Here's the drawing with two shaded views (mm, measured from the low corner). I have some questions. Give positions to 0.01 mm unless a question says otherwise; leave off trailing zeros. Write each loop counter-clockwise with the first axis right and the second up, starting at its lowest first coordinate (ties: lowest second). Pieces come first, ordered by that corner, then holes. Notation, with made-up numbers: M 29.25,79 L 62.25,79 A21 cw 62.25,84 Z; hole C 31.5,62.25 d5. An arc over 180 degrees is marked long. Use one line per item in the form item = value.
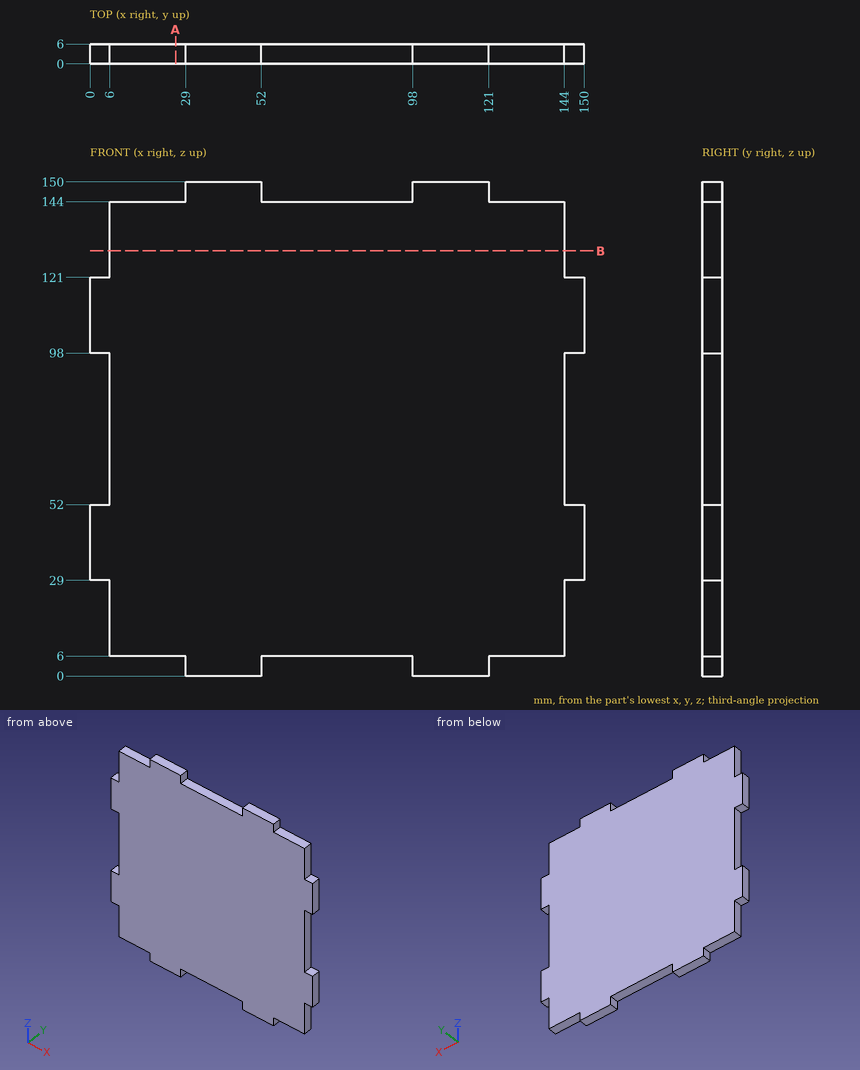
1) If I drill on L1, parallel to X at y = 2.85, z = 75.5, over which ranges is the centre line in solid material (lowest first)?
Checked values:
L1 = 6 to 144
2) For pin 1 Ø3 at (y, z) = (4, 137.5) entering from +X; pin 2 Ø3 at (x, y) = (147, 3.5) entering from -Z; pin 3 Ø1.8 at (x, y) = (148.5, 2.5) entering from +Z, each with a flat end and sliding along its axis, tell me the tip position at first contact or that it passes through.
Checked values:
pin_1 = 144
pin_2 = 29
pin_3 = 121
3) I want a section at B-B, the plane z = 129. Please give me the cut outline in (x, y).
Checked values:
outline = M 6,0 L 144,0 L 144,6 L 6,6 Z
4) I want a section at A-A, the plane x = 26. Please give me the cut outline in (y, z).
Checked values:
outline = M 0,6 L 6,6 L 6,144 L 0,144 Z
